Autodesk Inventor part; units mm, degrees
ref_plane "YZ Plane" through (0, 0, 0) normal (1, 0, 0) x (0, 1, 0)
ref_plane "XZ Plane" through (0, 0, 0) normal (0, 1, 0) x (-1, 0, 0)
ref_plane "XY Plane" through (0, 0, 0) normal (0, 0, 1) x (1, 0, 0)
sketch "Sketch1" plane through (0, 0, 0) normal (0, 0, 1) x (1, 0, 0)
  line L0 (0, 0) -> (-22.6274, 22.6274) construction
  circle A0 centre (0, 0) radius 32 construction
  line L1 (-31, 0) -> (-45, 0) construction
  line L2 (-45, 0) -> (-45, 19) construction
  line L3 (-45, 19) -> (-31, 19) construction
  line L4 (-31, 19) -> (-31, 0) construction
  line L5 (-31, 0) -> (0, 0) construction
  circle A1 centre (0, 0) radius 30 construction
  line L6 (-22.6274, 22.6274) -> (-0.7071, 44.5477)
  line L7 (-0.7071, 44.5477) -> (-2.1213, 45.9619)
  line L8 (-2.1213, 45.9619) -> (-24.0416, 24.0416)
  line L9 (-24.0416, 24.0416) -> (-22.6274, 22.6274)
  line L10 (-24.0416, 24.0416) -> (-22.6274, 22.6274)
  line L11 (-22.6274, 22.6274) -> (-25.4558, 19.799)
  line L12 (-25.4558, 19.799) -> (-26.8701, 21.2132)
  line L13 (-26.8701, 21.2132) -> (-24.0416, 24.0416)
  line L14 (-25.4558, 19.799) -> (-31, 19)
  line L15 (-31, 19) -> (-45, 19)
  line L16 (-45, 19) -> (-45, 24)
  line L17 (-45, 24) -> (-24.0833, 24)
  line L18 (-26.8701, 21.2132) -> (-24.0833, 24)
  line L19 (-0.7071, 44.5477) -> (0, 44.5477)
  line L20 (0, 44.5477) -> (0, 32)
  arc A2 (0, 32) -> (-22.6274, 22.6274) centre (0, 0) ccw
  point P0 (0, 38.2739)
  dimension "d0" = 19
  dimension "d1" = 31
  dimension "d2" = 14
  dimension "d4" = 60
  dimension "d5" = 2
  dimension "d6" = 2
  dimension "d8" = 4
  dimension "d9" = 35
  dimension "d10" = 45
  dimension "d13" = 5
extrude "Extrusion1" add sketch "Sketch1" along normal blind 21
sketch "Sketch2" plane through (-24.0833, 24, 0) normal (-0.7071068, 0.7071068, 0) x (-0.7071068, -0.7071068, 0)
  line L0 (-31.0589, 0) -> (-31.0589, 21) construction
  line L1 (-31.0589, 2) -> (-11.0589, 2)
  line L2 (-11.0589, 2) -> (-11.0589, 19)
  line L3 (-11.0589, 19) -> (-31.0589, 19)
  line L4 (-31.0589, 19) -> (-31.0589, 2)
  line L5 (-31.0589, 0) -> (0, 0) construction
  line L6 (-31.0589, 21) -> (0, 21) construction
  line L7 (-31.0589, 2) -> (-31.0589, 0)
  line L8 (0, 0) -> (0, 21)
  line L9 (-31.0589, 0) -> (0, 0)
  line L10 (0, 0) -> (0, 21)
  line L11 (0, 21) -> (-31.0589, 21)
  line L12 (-31.0589, 21) -> (-31.0589, 19)
  point P0 (-0.0589, 0)
  point P1 (-31.0589, 10.5)
  dimension "d14" = 17
  dimension "d15" = 20
extrude "Extrusion2" add sketch "Sketch2" along normal blind 5 contours L1 L2 L3 L12 L11 L8 L9 L7
sketch "Sketch3" plane through (-16.2635, 31.8198, 2) normal (0.7071068, 0.7071068, 0) x (-0.7071068, 0.7071068, 0)
  line L0 (0, 0) -> (0, 17) construction
  line L1 (0, 0) -> (5, 0) construction
  line L2 (5, 17) -> (5, 0) construction
  line L3 (0, 17) -> (5, 17) construction
  line L4 (5, 5.5) -> (0, 5.5)
  line L5 (0, 5.5) -> (0, 11.5)
  line L6 (0, 11.5) -> (5, 11.5)
  line L7 (5, 11.5) -> (5, 5.5)
  line L8 (0, 0) -> (0, 17)
  point P0 (-34, -2)
  point P1 (5, 8.5)
  point P2 (0, 8.5)
  dimension "d18" = 6
sketch "Sketch4" plane through (0, 0, 21) normal (0, 0, 1) x (1, 0, 0)
  line L0 (-24.0833, 24) -> (-45, 24)
  line L1 (-45, 24) -> (-45, 19)
  line L2 (-45, 19) -> (-31, 19)
  line L3 (-31, 19) -> (-25.4558, 19.799)
  line L4 (-25.4558, 19.799) -> (-22.6274, 22.6274)
  line L5 (-0.7071, 44.5477) -> (-5.6569, 49.4975)
  line L6 (-27.6188, 27.5355) -> (-5.6569, 49.4975)
  line L7 (-24.0833, 24) -> (-27.6188, 27.5355)
  line L8 (-11.3137, 43.8406) -> (-14.1421, 46.669)
  line L9 (-14.1421, 46.669) -> (-31, 29.8112)
  line L10 (-31, 29.8112) -> (-31, 24)
  arc A0 (0, 32) -> (-22.6274, 22.6274) centre (0, 0) ccw
  line L11 (0, 32) -> (0, 44.5477)
  line L12 (0, 44.5477) -> (-0.7071, 44.5477)
  dimension "d19" = 8
  dimension "d20" = 4
extrude "Extrusion3" add sketch "Sketch4" against normal up to surface (21 mm away) contours L0 L10 L9 L8 L6 L7
extrude "Extrusion4" cut sketch "Sketch3" against normal blind 17
sketch "Sketch5" plane through (-45, 24, 21) normal (0, 1, 0) x (1, 0, 0)
  line L0 (14, 0) -> (14, 7.5) construction
  line L1 (14, 21) -> (0, 21) construction
  line L2 (0, 21) -> (0, 0) construction
  line L3 (14, 0) -> (0, 0) construction
  line L4 (0, 21) -> (0, 0) construction
  line L5 (0, 10.5) -> (14, 10.5) construction
  line L6 (14, 0) -> (14, 21) construction
  line L7 (7, 16.5) -> (7, 4.5) construction
  circle A0 centre (7, 16.5) radius 2.5
  circle A1 centre (7, 4.5) radius 2.5
  line L8 (13.8457, 13.5) -> (14, 13.5)
  line L9 (14, 13.5) -> (14, 21)
  line L10 (14, 7.5) -> (13.8457, 7.5)
  line L11 (13.8457, 7.5) -> (13.8457, 13.5)
  point P0 (45, 21)
  point P1 (7, 10.5)
  dimension "d25" = 5
  dimension "d26" = 12
extrude "Extrusion5" cut sketch "Sketch5" against normal through all
properties part number "hall follower"
Check sheet for the modelled part. Datum: model origin and axes. Units: mm. A direction names the side the tool comes from. Round coordinates to 2 decimals unless told otherwise and drop trailing zeros. Loops run counter-clockwise (first coordinate to the right, second up) from the corner with the lowest first, then second, coordinate; pieces in that order, holes last. Notation, with made-up numbers: (85, -10.5) - (127, -10.5) arc R21 cw to (127, -4.5) - close; hole circle Ø4 at (-4.5, 19.25). An arc over 180 degrees is marked (long way). Answer as a JSON object with one key per item and string values. Group by question number.
Q1. Gauge pin test, flat ends, axial feed: P1, Ø0.6, axis at x = 0, z = 11, coming from the +Y side; P2, Ø6.5, axis at x = -38, z = 16.5, coming from the +Y side; P3, Ø8, axis at x = -14.5, z = 14.5, coming from the -Y side; P4, Ø4, axis at x = -27, y = 38, coming from the -Z side. Record the tip position at first contact, or that the pin passes through.
Q2. Mould release check, pull along Z, two halves, no side actions. Record for faces 6 (the face through (-8.446, 46.709, 20.014)), 7 (the face through (-11, 41, 2)): released by +Z, released by -Z, zero draft, split by the parting line, or undercut.
Q3. Sectioned sample at B-B, the plane z = 8.5. Enter the section's corners in (x, y), plus the area to 3 significant figures.
Q4. Sectioned sample at A-A, the plane x = -38. Enter the section's corners in (y, z).
Q5. Scan lines: line 1 along Z through (x, y) = (-38, 20.4); line 2 along Z through (x, y) = (-17.5, 34.5); line 3 along Y through (x, z) = (-34, 6.5). Record each from-to range of solid material in increasing order. Write a range as [from, to].
Q6. Sectioned sample at C-C, the plane x = -18. Enter the section's corners in (y, z), plus the area to 3 significant figures.
Q7. Set-up check for faces 1 (the face through (0, 38, 10)), 2 (the face through (-35.69, 21.54, 17.46)), 3 (the face through (-38, 24, 10)), 4 (the face through (-30.03, 21.54, 10.54)), 5 (the face through (-12.708, 45.235, 10.647)): record each of +Z, -Z, +X, -X, +Y, -Y from which the full face is reachable in a straight line by a thin tool's end or side.
Q8. Sectioned sample at D-D, the plane z = 4.5. Enter the section's corners in (x, y).
Solution:
{
 "1": {"P1": "stops at y = 44.55", "P2": "stops at y = 24", "P3": "stops at y = 26.11", "P4": "passes through"},
 "2": {"face 6": "zero draft", "face 7": "undercut"},
 "3": {"outline": "(-45, 19) - (-31, 19) - (-25.46, 19.8) - (-22.63, 22.63) arc R32 cw to (0, 32) - (0, 44.55) - (-0.71, 44.55) - (-2.12, 45.96) - (-28.29, 19.8) - (-31.82, 23.33) - (-31.15, 24) - (-45, 24) - close; (-31, 24.15) - (-19.8, 35.36) - (-11.31, 43.84) - (-14.14, 46.67) - (-31, 29.81) - close", "area": "360 mm²"},
 "4": {"outline": "(19, 0) - (24, 0) - (24, 2) - (19, 2) - close; (19, 7) - (24, 7) - (24, 14) - (19, 14) - close; (19, 19) - (24, 19) - (24, 21) - (19, 21) - close"},
 "5": {"line 1": "z = [0, 2], [7, 14], [19, 21]", "line 2": "z = [0, 2], [19, 21]", "line 3": "y = [19, 24]"},
 "6": {"outline": "(26.46, 0) - (42.81, 0) - (42.81, 21) - (26.46, 21) - close; hole (30.08, 7.5) - (33.56, 7.5) - (33.56, 2) - (37.15, 2) - (37.15, 19) - (33.56, 19) - (33.56, 13.5) - (30.08, 13.5) - close", "area": "261 mm²"},
 "7": {"face 1": "+Z, -Z, +X, +Y, -Y", "face 2": "+Y, -Y", "face 3": "+Z, -Z, -X, +Y", "face 4": "none", "face 5": "+Z, -Z, +Y"},
 "8": {"outline": "(-45, 19) - (-40.5, 19) - (-40.5, 24) - (-45, 24) - close; (-35.5, 19) - (-31, 19) - (-25.46, 19.8) - (-22.63, 22.63) arc R32 cw to (0, 32) - (0, 44.55) - (-0.71, 44.55) - (-2.12, 45.96) - (-16.26, 31.82) - (-19.8, 35.36) - (-11.31, 43.84) - (-14.14, 46.67) - (-31, 29.81) - (-31, 24) - (-35.5, 24) - close"}
}
